```python
from build123d import *

# Parameters (mm, degrees)
SKETCH1_R                = 0.85
BOSS_EXTRUDE1_DEPTH      = 6
BOSS_EXTRUDE2_DEPTH      = 9
BOSS_EXTRUDE2_DEPTH_BACK = 6
SKETCH4_R                = 1.25
CUT_EXTRUDE2_DEPTH       = 49.187135213
CUT_EXTRUDE3_DEPTH       = 10
SKETCH7_W                = 1.75
SKETCH7_H                = 1.78
BOSS_EXTRUDE4_DEPTH      = 6


with BuildPart() as part:
    # Sketch1 → Boss-Extrude1 (new body)
    with BuildSketch(Plane(origin=(0, 0, 0), x_dir=(1, 0, 0), z_dir=(0, 1, 0))):
        with BuildLine():
            Line((-17, -6.5), (-17, -33.5))
            Line((-17, -33.5), (-17, -39))
            Line((-17, -39), (17, -39))
            Line((17, -39), (17, -33.5))
            Line((17, -33.5), (17, -6.5))
            Line((17, -6.5), (15.25, -6.5))
            ThreePointArc((15.25, -6.5), (13.258096668, -9.951651759), (10.5, -12.828191611))
            Line((10.5, -12.828191611), (10.5, -30.5))
            Line((10.5, -30.5), (8, -30.5))
            Line((8, -30.5), (8, -33))
            Line((8, -33), (-8, -33))
            Line((-8, -33), (-8, -30.5))
            Line((-8, -30.5), (-10.5, -30.5))
            Line((-10.5, -30.5), (-10.5, -12.828191611))
            ThreePointArc((-10.5, -12.828191611), (-13.258096668, -9.951651759), (-15.25, -6.5))
            Line((-15.25, -6.5), (-17, -6.5))
        make_face()
        with Locations(Location((-13.5, -30.5, 0), (0, 0, 270))):
            Circle(SKETCH1_R, mode=Mode.SUBTRACT)
        with Locations(Location((-13.5, -22.5, 0), (0, 0, 270))):
            Circle(SKETCH1_R, mode=Mode.SUBTRACT)
        with Locations(Location((-13.5, -14.5, 0), (0, 0, 270))):
            Circle(SKETCH1_R, mode=Mode.SUBTRACT)
        with Locations(Location((-8, -36, 0), (0, 0, 270))):
            Circle(SKETCH1_R, mode=Mode.SUBTRACT)
        with Locations(Location((8, -36, 0), (0, 0, 270))):
            Circle(SKETCH1_R, mode=Mode.SUBTRACT)
        with Locations(Location((13.5, -30.5, 0), (0, 0, 270))):
            Circle(SKETCH1_R, mode=Mode.SUBTRACT)
        with Locations(Location((13.5, -22.5, 0), (0, 0, 270))):
            Circle(SKETCH1_R, mode=Mode.SUBTRACT)
        with Locations(Location((13.5, -14.5, 0), (0, 0, 270))):
            Circle(SKETCH1_R, mode=Mode.SUBTRACT)
    extrude(amount=BOSS_EXTRUDE1_DEPTH)

    # Sketch3 → Boss-Extrude2 (add, two sides: drawn at the far end of the back side and taken through both)
    with BuildSketch(Plane.XZ.offset(-BOSS_EXTRUDE2_DEPTH_BACK)):
        Polygon((17, 22.74), (24, 22.74), (24, 4.72), (17, 4.72), (17, 7.901808389), align=None)
    extrude(amount=BOSS_EXTRUDE2_DEPTH + BOSS_EXTRUDE2_DEPTH_BACK)

    # Sketch4 → Cut-Extrude2 (cut, through all)
    with BuildSketch(Plane.XZ.offset(9)):
        with Locations(Location((20.5, 7.63, 0), (0, 0, 270))):
            Circle(SKETCH4_R)
        with Locations(Location((20.5, 13.59, 0), (0, 0, 270))):
            Circle(SKETCH4_R)
        with Locations(Location((20.5, 19.69, 0), (0, 0, 270))):
            Circle(SKETCH4_R)
    extrude(amount=-CUT_EXTRUDE2_DEPTH, mode=Mode.SUBTRACT)

    # Sketch5 → Cut-Extrude3 (cut)
    with BuildSketch(Plane.XZ):
        with BuildLine():
            Line((8, 33), (-8, 33))
            ThreePointArc((-8, 33), (-9.767766953, 32.267766953), (-10.5, 30.5))
            Line((-10.5, 30.5), (10.5, 30.5))
            ThreePointArc((10.5, 30.5), (9.767766953, 32.267766953), (8, 33))
        make_face()
    extrude(amount=-CUT_EXTRUDE3_DEPTH, mode=Mode.SUBTRACT)

    # Sketch7 → Boss-Extrude4 (add)
    with BuildSketch(Plane(origin=(0, 6, 0), x_dir=(1, 0, 0), z_dir=(0, 1, 0))):
        with Locations((16.125, -5.61)):
            Rectangle(SKETCH7_W, SKETCH7_H)
    extrude(amount=-BOSS_EXTRUDE4_DEPTH)


solid = part.part
```
Geometry: final body of the model. Coordinates: model frame, mm. A direction names the side the tool comes from. Coordinates: 2 decimals unless noted, no trailing zeros. Loops run counter-clockwise (first coordinate to the right, second up) from the corner with the lowest first, then second, coordinate; pieces in that order, holes last. Notation, with made-up numbers: (38.5, -27) -> (79.5, -27) arc R28 cw to (79.5, -9) -> close; hole circle Ø8 at (81, 86). An arc over 180 degrees is marked (long way). Use a Markdown table: item, result. Add a question column.
(1) Mould query, pull axis X, two halves, no side actions, for faces 4 (the flat face through (17, -4, 14)), 5 (the flat face through (0, 3, 39)), 6 (the cylindrical face through (-13.22, 2.96, 10)). Classes: pulls with the +X half, pulls with the -X half, needs draft (parallel to the pull), parting line crosses it, or undercut.
(2) Line query: line 1 along X through (y, z) = (4.75, 22.5); line 2 along X through (y, z) = (1.35, 36); line 3 along Z through (x, y) = (21.5, -7.25). Output: solid intervals per line, ascending.
(3) Pin query (flat end, axial travel): pin 1 Ø3 at (x, z) = (20.5, 13.59) entering from -Y; pin 2 Ø1.5 at (x, y) = (5, 1.5) entering from -Z; pin 3 Ø2.5 at (x, z) = (13.5, 14.5) entering from -Y; pin 4 Ø5 at (y, z) = (-4, 18.5) entering from -X. Return the tip coordinate at first contact, or that it passes through.
(4) Section query D-D, the plane y = -7.75. Return loops of the section in (x, z), plus the area to 3 significant figures.
(5) Section query B-B, the plane z = 36. Return loops of the section in (x, y).
(6) Access query for faces 1 (the flat face through (-16, 3, 6.5)), 2 (the flat face through (0, 3, 33)), 3 (the cylindrical face through (-13.46, 2.96, 29.65)). Directions: +Z, -Z, +X, -X, +Y, -Y. A direction counts if a zero-diameter tool reaches every point of the face in a straight line with its end or side. Return the directions, or none.
(7) Section query C-C, the plane y = 3.75. State how many separate pieces and enclosed holes the cut face has, plus the area to 3 significant figures.
(8) Section query A-A, the plane z = 28. Return loops of the section in (x, y), plus the area to 3 significant figures.
Answer:
| question | item | result |
|---|---|---|
| 1 | face 4 | pulls with the -X half |
| 1 | face 5 | needs draft |
| 1 | face 6 | undercut |
| 2 | line 1 | x = -17 to -14.35, -12.65 to -10.5, 10.5 to 12.65, 14.35 to 24 |
| 2 | line 2 | x = -17 to -8.85, -7.15 to 7.15, 8.85 to 17 |
| 2 | line 3 | z = 4.72 to 6.88, 8.38 to 12.84, 14.34 to 18.94, 20.44 to 22.74 |
| 3 | pin 1 | stops at y = -9 |
| 3 | pin 2 | stops at z = 33 |
| 3 | pin 3 | stops at y = 0 |
| 3 | pin 4 | stops at x = 17 |
| 4 | outline | (17, 4.72) -> (24, 4.72) -> (24, 22.74) -> (17, 22.74) -> close; hole circle Ø2.5 at (20.5, 7.63); hole circle Ø2.5 at (20.5, 13.59); hole circle Ø2.5 at (20.5, 19.69) |
| 4 | area | 111 mm^2 |
| 5 | outline | (-17, 0) -> (-8.85, 0) -> (-8.85, 6) -> (-17, 6) -> close; (-7.15, 0) -> (7.15, 0) -> (7.15, 6) -> (-7.15, 6) -> close; (8.85, 0) -> (17, 0) -> (17, 6) -> (8.85, 6) -> close |
| 6 | face 1 | -Z, -X, +Y, -Y |
| 6 | face 2 | -Z, +Y, -Y |
| 6 | face 3 | +Y, -Y |
| 7 | separate pieces | 1 |
| 7 | enclosed holes | 11 |
| 7 | area | 612 mm^2 |
| 8 | outline | (-17, 0) -> (-10.5, 0) -> (-10.5, 6) -> (-17, 6) -> close; (10.5, 0) -> (17, 0) -> (17, 6) -> (10.5, 6) -> close |
| 8 | area | 78.0 mm^2 |
